from build123d import *

# Parameters (mm, degrees)
BOSS_EXTRUDE1_DEPTH = 30
SKETCH2_R           = 1.65
CUT_EXTRUDE2_DEPTH  = 30
FILLET1_R           = 5
FILLET2_R           = 1


with BuildPart() as part:
    # Sketch1 → Boss-Extrude1 (new body)
    with BuildSketch(Plane.XY):
        Polygon((-13.25, -40.4), (-13.25, -25.4), (13.25, -25.4), (13.25, 25.4), (-13.25, 25.4), (-13.25, 40.4), (-8.25, 40.4), (-8.25, 30.4), (18.25, 30.4), (18.25, -30.4), (-8.25, -30.4), (-8.25, -40.4), align=None)
    extrude(amount=BOSS_EXTRUDE1_DEPTH)

    # Sketch2 → Cut-Extrude2 (cut)
    with BuildSketch(Plane.ZY.offset(13.25)):
        with Locations((7, 34.4)):
            Circle(SKETCH2_R)
        with Locations((23, 34.4)):
            Circle(SKETCH2_R)
        with Locations((7, -34.4)):
            Circle(SKETCH2_R)
        with Locations((23, -34.4)):
            Circle(SKETCH2_R)
    extrude(amount=-CUT_EXTRUDE2_DEPTH, mode=Mode.SUBTRACT)

    # Fillet1
    fillet1_edges = [part.edges().sort_by_distance(p)[0] for p in [
        (18.25, 30.4, 15),
        (18.25, -30.4, 15),
    ]]
    fillet(fillet1_edges, radius=FILLET1_R)

    # Fillet2
    fillet2_edges = [part.edges().sort_by_distance(p)[0] for p in [
        (-8.25, 40.4, 15),
        (-8.25, 30.4, 15),
        (-8.25, -30.4, 15),
        (-8.25, -40.4, 15),
    ]]
    fillet(fillet2_edges, radius=FILLET2_R)


solid = part.part
Model file for the job. Use its own axes, mm. A direction names the side the tool comes from. Give positions to 0.01 mm unless a question says otherwise; leave off trailing zeros. Write each loop counter-clockwise with the first axis right and the second up, starting at its lowest first coordinate (ties: lowest second). Pieces come first, ordered by that corner, then holes. Notation, with made-up numbers: (2, 42) - (41, 42) arc R33 cw to (41, 80) - close; hole circle Ø8 at (68, -7.75). An arc over 180 degrees is marked (long way). Answer as CSV lines item,"result".
1. Band-saw the part on A-A (x = 5). Write the cut outline in (y, z), and give its area (3 significant figures).
Responses:
outline,"(-30.4, 0) - (-25.4, 0) - (-25.4, 30) - (-30.4, 30) - close; (25.4, 0) - (30.4, 0) - (30.4, 30) - (25.4, 30) - close"
area,"300 mm2"
2. Drill centre lines: L1, parallel to Y at x = -9.45, z = 23; L2, parallel to Z at x = -11, y = 34; L3, parallel to Y at x = 5.5, z = 24.5. Where is each one in solid material? Low to high. Write a range as [from, to].
Responses:
L1,"y = [-40.4, -36.05], [-32.75, -25.4], [25.4, 32.75], [36.05, 40.4]"
L2,"z = [0, 5.4], [8.6, 21.4], [24.6, 30]"
L3,"y = [-30.4, -25.4], [25.4, 30.4]"
3. Band-saw the part on D-D (z = 4.25). Write the cut outline in (x, y).
Responses:
outline,"(-13.25, -40.4) - (-9.25, -40.4) arc R1 ccw to (-8.25, -39.4) - (-8.25, -31.4) arc R1 cw to (-7.25, -30.4) - (13.25, -30.4) arc R5 ccw to (18.25, -25.4) - (18.25, 25.4) arc R5 ccw to (13.25, 30.4) - (-7.25, 30.4) arc R1 cw to (-8.25, 31.4) - (-8.25, 39.4) arc R1 ccw to (-9.25, 40.4) - (-13.25, 40.4) - (-13.25, 25.4) - (13.25, 25.4) - (13.25, -25.4) - (-13.25, -25.4) - close"
4. Two-plate mould, pull along Y, no slides. Class faces 1 (the face through (16.82, -28.9, 15.21)), 2 (the face through (18.25, 0, 15)), 3 (the face through (13.25, 0, 15)), 4 (the face through (3, 30.4, 15)): +Y half, -Y half, draft (parallel to the pull), parting line (faces both ways), or undercut.
Responses:
face 1,"-Y half"
face 2,"draft"
face 3,"undercut"
face 4,"+Y half"
5. 3-axis set-ups, long thin cutter, end or side, ignore diameter. For faces 5 (the face through (0, -25.4, 15)), 6 (the face through (-8.25, 35, 15)), 7 (the face through (-11, 40.4, 15)), 8 (the face through (3, -30.4, 15)), 9 (the face through (-13.25, 33, 15)): which of +Z, -Z, +X, -X, +Y, -Y reach the whole face in a straight line?
Responses:
face 5,"+Z, -Z, -X"
face 6,"+Z, -Z, +X, +Y"
face 7,"+Z, -Z, +X, -X, +Y"
face 8,"+Z, -Z, +X, -Y"
face 9,"+Z, -Z, -X, +Y, -Y"
6. Band-saw the part on C-C (y = 34.4). Write the cut outline in (x, z), and give its area (3 significant figures).
Responses:
outline,"(-13.25, 0) - (-8.25, 0) - (-8.25, 5.35) - (-13.25, 5.35) - close; (-13.25, 8.65) - (-8.25, 8.65) - (-8.25, 21.35) - (-13.25, 21.35) - close; (-13.25, 24.65) - (-8.25, 24.65) - (-8.25, 30) - (-13.25, 30) - close"
area,"117 mm2"
7. Pin check, flat tips, straight feed: pin 1 (3 mm diameter, centred on y = 34.4, z = 7, fed in from +X); pin 2 (13 mm diameter, centred on x = 5, z = 15.5, fed in from -Y); pin 3 (8 mm diameter, centred on x = 0, z = 12, fed in from +Y); pin 4 (4 mm diameter, centred on y = -33.5, z = 14, fed in from +X). Stop position of each tip, or through.
Responses:
pin 1,"passes through"
pin 2,"stops at y = -30.4"
pin 3,"stops at y = 30.4"
pin 4,"stops at x = -8.25"
8. Band-saw the part on B-B (z = 23). Write the cut outline in (x, y), and give its area (3 significant figures).
Responses:
outline,"(-13.25, -40.4) - (-9.25, -40.4) arc R1 ccw to (-8.25, -39.4) - (-8.25, -36.05) - (-13.25, -36.05) - close; (-13.25, -32.75) - (-8.25, -32.75) - (-8.25, -31.4) arc R1 cw to (-7.25, -30.4) - (13.25, -30.4) arc R5 ccw to (18.25, -25.4) - (18.25, 25.4) arc R5 ccw to (13.25, 30.4) - (-7.25, 30.4) arc R1 cw to (-8.25, 31.4) - (-8.25, 32.75) - (-13.25, 32.75) - (-13.25, 25.4) - (13.25, 25.4) - (13.25, -25.4) - (-13.25, -25.4) - close; (-13.25, 36.05) - (-8.25, 36.05) - (-8.25, 39.4) arc R1 ccw to (-9.25, 40.4) - (-13.25, 40.4) - close"
area,"625 mm2"
